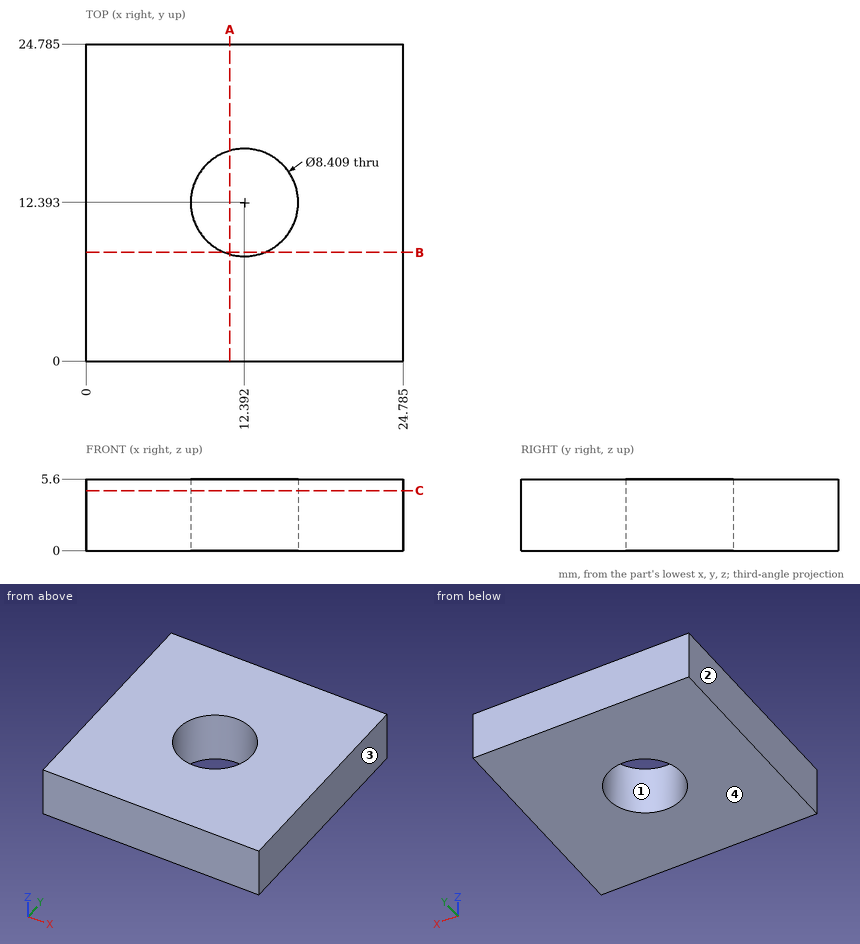
Answer from the drawing. Dimensions are ordinates in mm from the lowest x, y and z of the part. Give positions to 0.01 mm unless a question says otherwise; leave off trailing zeros. Loops run counter-clockwise (first coordinate to the right, second up) from the corner with the lowest first, then second, coordinate; pieces in that order, holes last.
Item 1: Determine the mould class of the marked faces 1, 2, 3 and 4 for opening direction X: +X half, -X half, draft (parallel to the pull), parting line (faces both ways), or undercut.
Derived:
face 1: undercut
face 2: -X half
face 3: +X half
face 4: draft
Item 2: A cutting plane is placed at B-B (y = 8.5). Give the vertices of the cut face in (x, z) (1 decimal).
Derived:
outline: (0, 0) - (10.8, 0) - (10.8, 5.6) - (0, 5.6) - close; (14, 0) - (24.8, 0) - (24.8, 5.6) - (14, 5.6) - close
Item 3: A cutting plane is placed at A-A (x = 11.25). Give the vertices of the cut face in (y, z) (1 decimal).
Derived:
outline: (0, 0) - (8.3, 0) - (8.3, 5.6) - (0, 5.6) - close; (16.4, 0) - (24.8, 0) - (24.8, 5.6) - (16.4, 5.6) - close
Item 4: Find the intervals of material crossed by line 1 along Y through (x, z) = (15, 3.1) (1 decimal); line 2 along Y through (x, z) = (13.75, 4.3) (1 decimal); line 3 along X through (y, z) = (15.5, 2.1) (1 decimal), in increasing order.
Derived:
line 1: y = 0 to 9.1, 15.7 to 24.8
line 2: y = 0 to 8.4, 16.4 to 24.8
line 3: x = 0 to 9.6, 15.2 to 24.8
Item 5: A cutting plane is placed at C-C (z = 4.7). Give the vertices of the cut face in (x, y) (1 decimal).
Derived:
outline: (0, 0) - (24.8, 0) - (24.8, 24.8) - (0, 24.8) - close; hole circle Ø8.4 at (12.4, 12.4)
